```python
from build123d import *

# Parameters (mm, degrees)
F0_R      = 22.1
F2_R      = 18.1
F7_FACE_R = 18.1
F4_R      = 18.1
F8_FACE_R = 18.1
F6_R      = 24.1


with BuildPart() as f7:
    # F0 (on Top) → F7 section 0
    with BuildSketch(Plane.XY):
        Circle(F0_R)
    # F2 (on offset) → F7 section 1
    with BuildSketch(Plane.XY.offset(5)):
        Circle(F2_R)
    loft()

    # F7_face (on face) → F8 section 0
    with BuildSketch(Plane.XY.offset(5)):
        Circle(F7_FACE_R)
    # F4 (on offset) → F8 section 1
    with BuildSketch(Plane.XY.offset(155)):
        Circle(F4_R)
    loft()

    # F8_face (on face) → F9 section 0
    with BuildSketch(Plane.XY.offset(155)):
        Circle(F8_FACE_R)
    # F6 (on offset) → F9 section 1
    with BuildSketch(Plane.XY.offset(160)):
        Circle(F6_R)
    loft()


solid = f7.part
```
Read the model definition and answer for the solid it produces. Units are mm, in the model's axes. Round coordinates to 2 decimals unless told otherwise and drop trailing zeros. Write each loop counter-clockwise with the first axis right and the second up, starting at its lowest first coordinate (ties: lowest second). Pieces come first, ordered by that corner, then holes. Notation, with made-up numbers: (86, -4.5) - (145, -4.5) arc R7 ccw to (145, 6.5) - close; hole circle Ø1 at (-8, 88). An arc over 180 degrees is marked (long way). One line per item, written item: value.
Q1. For a pull along Z with two mould halves and no side action, classify faces 1 (the cylindrical face through (17.264, 5.437, 81.05)), 2 (the conical face through (-4.005, -18.036, 155.313)), 3 (the flat face through (0, 0, 160)), 4 (the flat face through (0, 0, 0)) as pulls with the +Z half, pulls with the -Z half, needs draft (parallel to the pull), parting line crosses it, or undercut.
The answers:
face 1: undercut
face 2: undercut
face 3: pulls with the +Z half
face 4: pulls with the -Z half
Q2. Each of these flat-tipped pins is pushed along its axis until it touches: P1, Ø3, axis at x = -4.5, z = 21.5, coming from the +Y side; P2, Ø1, axis at y = 1.5, z = 19.5, coming from the +X side; P3, Ø12, axis at x = 9.5, y = 7.5, coming from the -Z side; P4, Ø3, axis at x = -8.5, z = 23.5, coming from the -Y side. Where does it stop, or does it pass through?
The answers:
P1: stops at y = 17.85
P2: stops at x = 18.07
P3: stops at z = 0
P4: stops at y = -16.69
Q3. Find section A-A (x = 0). Determine the outline of the cut face in (y, z), and give its area (3 significant figures).
The answers:
outline: (-24.1, 160) - (-18.1, 155) - (-18.1, 5) - (-22.1, 0) - (22.1, 0) - (18.1, 5) - (18.1, 155) - (24.1, 160) - close
area: 5,840 mm2
Q4. Find section B-B (z = 31). Determine the outline of the cut face in (x, y).
The answers:
outline: circle Ø36.2 at (0, 0)
Q5. Straight lines are drawn through the part: line 1 (Z direction, x = 5, y = 17.5); line 2 (X direction, y = -1, z = 137); line 3 (Z direction, x = -13, y = 13.5). For each, find the intervals that lie inside material, in ascending order. Write a range as from..to.
The answers:
line 1: z = 0..4.87, 155.08..160
line 2: x = -18.07..18.07
line 3: z = 0..4.2, 155.53..160
